The figure shows three views and two pictorial views of one solid part (mm, origin at its lowest corner). Answer the questions. Coordinates: 2 decimals unless noted, no trailing zeros.
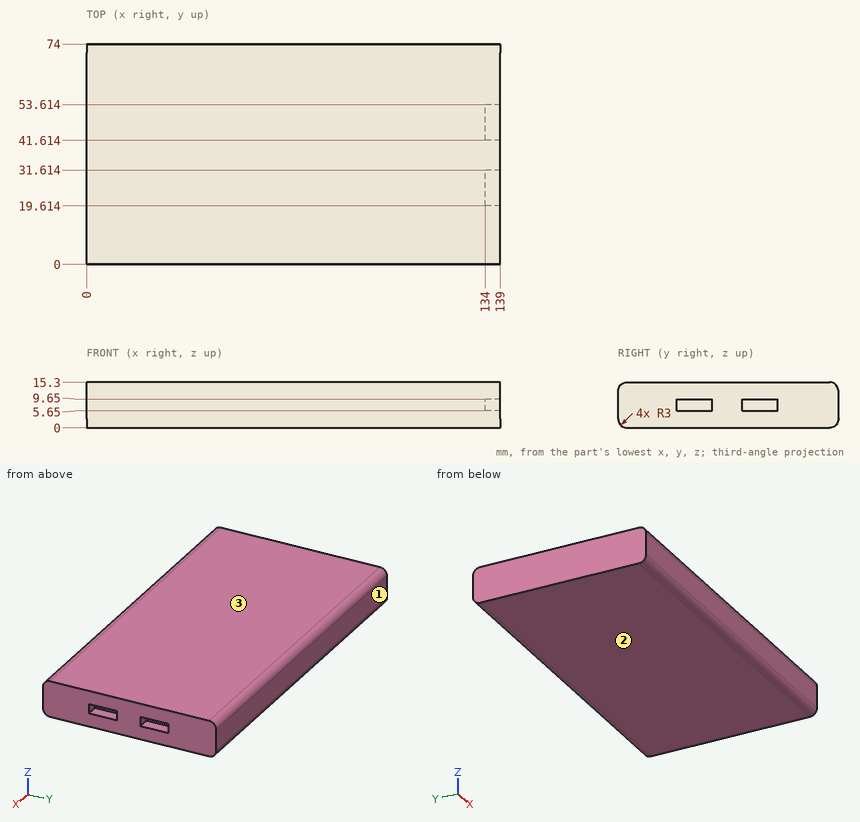
1) Straight lines are drawn through the part: probe 1 along X at (y, z) = (21, 6.5); probe 2 along Y at (x, z) = (98, 13.5); probe 3 along Y at (x, z) = (110, 1.25). For each, find the intervals that lie inside material, in ascending order.
2) This flat-tipped pin is pushed along its axis until it touches: P1, Ø1.2, axis at y = 49, z = 7, coming from the +X side. Where does it stop, or does it pass through?
3) The mould has two halves that part along Z. Classify the marked faces 1, 2 and 3: released by +Z, released by -Z, zero draft, split by the parting line, or undercut.
Working result:
1. probe 1: x = 0 to 134
1. probe 2: y = 0.25 to 73.75
1. probe 3: y = 0.56 to 73.44
2. P1: stops at x = 134
3. face 1: zero draft
3. face 2: released by -Z
3. face 3: released by +Z
